CAD build for the part. Positions are in the model's coordinates, mm. A direction names the side the tool comes from. Give positions to 0.01 mm unless a question says otherwise; leave off trailing zeros. Write each loop counter-clockwise with the first axis right and the second up, starting at its lowest first coordinate (ties: lowest second). Pieces come first, ordered by that corner, then holes. Notation, with made-up numbers: (-28.5, 76.5) - (-10.5, 76.5) arc R20 ccw to (-10.5, 111.5) - close; hole circle Ø7 at (-32, -37.75). An arc over 180 degrees is marked (long way). Write item = value, one per line. Start each with the question number.
Solid Edge part; units mm, degrees
sketch "Sketch1" plane through (0, 0, 0) normal (0, -1, 0) x (1, 0, 0)
  line L0 (2.5, 0) -> (5, 2.5)
  line L1 (5, 2.5) -> (5, 2.8)
  line L2 (5, 2.8) -> (0, 2.8)
  line L3 (0, 2.8) -> (0, -5.2)
  line L4 (0, -5.2) -> (2.0095, -5.2)
  line L5 (2.0095, -5.2) -> (2.5, -4.7095)
  line L6 (2.5, -4.7095) -> (2.5, -2.4)
  line L7 (2.5, -2.4) -> (2.0095, -2.4)
  line L8 (2.0095, -2.4) -> (2.0095, -2.39)
  line L9 (2.0095, -2.39) -> (2.5, -2.39)
  line L10 (2.5, -2.39) -> (2.5, 0)
  dimension "D1" = 2.5
  dimension "D2" = 2.0095
revolve "RevolvedProtrusion1" add sketch "Sketch1" angle 360 about axis through (0, 0, 54) along (0, 0, -1)
sketch "Sketch2" plane through (0, 0, 0) normal (0, -1, 0) x (1, 0, 0)
  arc A0 (-1.5, 0.5) -> (0, 0) centre (0, 2.5) ccw
  line L0 (0, 0.5) -> (0, 0)
  line L1 (-1.5, 0.5) -> (0, 0.5)
revolve "RevolvedCutout1" cut sketch "Sketch2" angle 360 about axis through (0, 0, 54) along (0, 0, -1)
sketch "Sketch3" plane through (0, 0, 2.8) normal (0, 0, 1) x (0, -1, 0)
  line L0 (-1.7321, 0) -> (-0.866, 1.5)
  line L1 (-0.866, 1.5) -> (0.866, 1.5)
  line L2 (0.866, 1.5) -> (1.7321, 0)
  line L3 (1.7321, 0) -> (0.866, -1.5)
  line L4 (0.866, -1.5) -> (-0.866, -1.5)
  line L5 (-0.866, -1.5) -> (-1.7321, 0)
extrude "Cutout1" cut sketch "Sketch3" against normal blind 2.3
cosmetic_thread "Thread1"
sketch "Sketch4" plane through (0, 0, 0) normal (1, 0, 0) x (0, 1, 0)
  line L0 (-1.72, 2.8) -> (0, 1.807)
revolve "RevolvedCutout2" cut sketch "Sketch4" angle 360 about axis through (0, 0, -57) along (0, 0, 1) material side at (0, -0.835, 2.3468)
fillet "Round1" radius 0.2 1 edges at (-2.5, 0, 0)
properties material "Stahl"
1. Mould opens along Y. For faces 4 (the cylindrical face through (-0.54, -2.44, -3.54)), 5 (the flat face through (2, 0, 2.8)), 6 (the flat face through (0.74, 1.305, 1.666)) say: +Y half, -Y half, draft (parallel to the pull), parting line (faces both ways), or undercut.
2. Cut at B-B (z = -4.5). Give the cut face in (x, y).
3. Cut at A-A (z = 2). Give the cut face in (x, y).
4. Tool access for faces 1 (the cylindrical face through (-0.54, -2.44, -1.22)), 2 (the flat face through (0, 0, -5.2)), 3 (the flat face through (-1.5, 0, 2)): list every direction of +Z, -Z, +X, -X, +Y, -Y with a clear straight run to the whole face (end or side of a thin tool).
5. Pin check, flat tips, straight feed: pin 1 Ø0.5 at (y, z) = (0.5, 2) entering from -X; pin 2 Ø4 at (y, z) = (0.5, -3.5) entering from -X; pin 3 Ø3 at (y, z) = (0, 0.5) entering from -X. Stop position of each tip, or through.
6. Wall check: line 1 along Y through (x, z) = (2, -1.25); line 2 along X through (y, z) = (-1, 1.25). Give the ranges that are in metal, low to high.
Output:
q1.face_4 = parting line
q1.face_5 = draft
q1.face_6 = undercut
q2.outline = circle Ø5 at (0, 0)
q3.outline = circle Ø9 at (0, 0); hole (-1.5, -0.87) - (0, -1.73) - (1.5, -0.87) - (1.5, 0.87) - (0, 1.73) - (-1.5, 0.87) - close
q4.face_1 = -Z
q4.face_2 = -Z, +X, -X, +Y, -Y
q4.face_3 = +Z
q5.pin_1 = -4.72
q5.pin_2 = -2.5
q5.pin_3 = -4.5
q6.line_1 = -1.5 to 1.5
q6.line_2 = -3.61 to -1.27, 1.27 to 3.61
